Autodesk Inventor part; units mm, degrees
ref_plane "YZ Plane" through (0, 0, 0) normal (1, 0, 0) x (0, 1, 0)
ref_plane "XZ Plane" through (0, 0, 0) normal (0, 1, 0) x (-1, 0, 0)
ref_plane "XY Plane" through (0, 0, 0) normal (0, 0, 1) x (1, 0, 0)
sketch "Sketch1" plane through (0, 0, 0) normal (0, 0, 1) x (1, 0, 0)
  line L0 (-12.245, 11.65) -> (-12.245, 3)
  line L1 (-12.245, 3) -> (-45.245, 3)
  line L2 (-45.245, 3) -> (-45.245, 0)
  line L3 (-45.245, 0) -> (-10.245, 0)
  line L4 (-10.245, 0) -> (-10.245, 8.8)
  line L5 (-10.245, 8.8) -> (10.245, 8.8)
  line L6 (10.245, 8.8) -> (10.245, 0)
  line L7 (10.245, 0) -> (45.245, 0)
  line L8 (45.245, 0) -> (45.245, 3)
  line L9 (45.245, 3) -> (12.245, 3)
  line L10 (12.245, 3) -> (12.245, 11.65)
  line L11 (12.245, 11.65) -> (-12.245, 11.65)
  line L12 (-10.245, 0) -> (10.245, 0) construction
  point P0 (0, 0)
  point P1 (0, 11.65)
  point P2 (0, 0)
  point P3 (-12.245, 7.325)
  point P4 (12.245, 7.325)
  dimension "d0" = 20.49
  dimension "d1" = 2.85
  dimension "d3" = 5.8
  dimension "d4" = 3
  dimension "d5" = 3
  dimension "d6" = 35
  dimension "d7" = 35
  dimension "d73" = 33
  dimension "d74" = 33
extrude "Extrusion1" add sketch "Sketch1" along normal mid plane 41.1
sketch "Sketch8" plane through (12.245, 3, 20.55) normal (0, 1, 0) x (1, 0, 0)
  line L0 (0, 41.1) -> (0, 0)
  line L1 (33, 0) -> (0, 0)
  line L2 (33, 41.1) -> (33, 0)
  line L3 (0, 41.1) -> (33, 41.1)
  line L4 (-57.49, 41.1) -> (-57.49, 0)
  line L5 (-24.49, 0) -> (-57.49, 0)
  line L6 (-24.49, 0) -> (-24.49, 41.1)
  line L7 (-57.49, 41.1) -> (-24.49, 41.1)
  line L8 (33, 41.1) -> (33, 0)
  circle A0 centre (-11.645, 30.6) radius 6.4
  line L9 (-12.245, 41) -> (-12.245, 0) construction
  point P0 (-12.245, 20.55)
  point P1 (-54.49, 30.65)
  point P2 (-29.49, 30.65)
  point P3 (-57.49, 20.55)
  point P4 (30, 30.65)
  point P5 (5, 30.65)
  dimension "d42" = 3
  dimension "d43" = 25
  dimension "d51" = 10.45
  dimension "d53" = 3
hole "Hole1" at (-42.245, 3, -10.1) at (-17.245, 3, -10.1) at (17.245, 3, -10.1) at (42.245, 3, -10.1) direction (0, -1, 0) diameter 2.53 end through all
sketch "Sketch9" plane through (12.245, 3, 20.55) normal (0, 1, 0) x (1, 0, 0)
  circle A0 centre (30, 30.65) radius 1.265
  circle A1 centre (5, 30.65) radius 1.265
  line L0 (0, 41.1) -> (0, 0)
  line L1 (33, 0) -> (0, 0)
  line L2 (33, 41.1) -> (33, 0)
  line L3 (0, 41.1) -> (33, 41.1)
  arc A2 (33, 24) -> (9, 0) centre (33, 0) ccw
  point P0 (-12.245, 20.55)
  dimension "d60" = 24
extrude "Extrusion2" cut sketch "Sketch9" against normal blind 10 contours A2 L2 L1
mirror "Mirror1" about plane through (0, 0, 0) normal (1, 0, 0) of "Extrusion2"
sketch "Sketch10" plane through (-12.245, 11.65, 20.55) normal (0, 1, 0) x (1, 0, 0)
  circle A0 centre (12.245, 30.602) radius 6.5
  line L0 (0, 41.1) -> (0, 0)
  line L1 (24.49, 0) -> (0, 0)
  line L2 (24.49, 41.1) -> (24.49, 0)
  line L3 (0, 41.1) -> (24.49, 41.1)
  point P0 (12.245, 20.55)
  point P1 (12.245, 41.1)
  dimension "d75" = 13
  dimension "d76" = 10.498
extrude "Extrusion3" cut sketch "Sketch10" against normal blind 10 contours A0
sketch "Sketch11" plane through (-12.245, 11.65, 20.55) normal (0, 1, 0) x (1, 0, 0)
  circle A0 centre (5.245, 10.482) radius 0.7835
  circle A1 centre (4.245, 23.702) radius 0.7835
  circle A2 centre (4.175, 38.602) radius 0.7835
  circle A3 centre (20.315, 38.602) radius 0.7835
  circle A4 centre (20.245, 23.702) radius 0.7835
  circle A5 centre (19.245, 10.482) radius 0.7835
hole "Hole2" at (-8, 11.65, -3.152) at (8, 11.65, -3.152) at (8.07, 11.65, -18.052) at (-8.07, 11.65, -18.052) at (-7, 11.65, 10.068) at (7, 11.65, 10.068) direction (0, -1, 0) diameter 2.1 end through all counterbore diameter 4.1 counterbore depth 1.4
fillet "Fillet3" radius 3 6 edges at (45.245, 1.5, -20.55) (45.245, 1.5, -3.45) (21.245, 1.5, 20.55) (-21.245, 1.5, 20.55) (-45.245, 1.5, -3.45) (-45.245, 1.5, -20.55)
sketch "Sketch15" plane through (-10.245, 8.8, 20.55) normal (0, -1, 0) x (1, 0, 0)
  line L0 (0, -41.1) -> (0, 0)
  line L1 (20.49, -41.1) -> (20.49, 0)
  line L2 (0, -41.1) -> (0, -44.1)
  line L3 (0, -44.1) -> (20.49, -44.1)
  line L4 (20.49, -44.1) -> (20.49, -41.1)
  line L5 (0, 0) -> (0, 3)
  line L6 (0, 3) -> (20.49, 3)
  line L7 (20.49, 3) -> (20.49, 0)
  line L8 (0, -44.1) -> (0, 3)
  line L9 (20.49, 3) -> (20.49, -44.1)
  point P0 (10.245, -20.55)
  point P1 (0, 1.5)
  dimension "d126" = 3
  dimension "d127" = 3
sketch "Sketch16" plane through (-12.245, 11.65, 20.55) normal (0, 1, 0) x (1, 0, 0)
  line L0 (-30, 41.1) -> (0, 41.1)
  arc A0 (-30, 41.1) -> (-33, 38.1) centre (-30, 38.1) ccw
  line L1 (-33, 38.1) -> (-33, 26.8328)
  arc A1 (-33, 26.8328) -> (-30.3333, 23.8514) centre (-30, 26.8328) ccw
  arc A2 (-9.1486, 2.6667) -> (-30.3333, 23.8514) centre (-33, 0) ccw
  arc A3 (-9.1486, 2.6667) -> (-6.1672, 0) centre (-6.1672, 3) ccw
  line L2 (0, 0) -> (-6.1672, 0)
  line L3 (24.49, 0) -> (0, 0)
  line L4 (30.6572, 0) -> (24.49, 0)
  arc A4 (30.6572, 0) -> (33.6386, 2.6667) centre (30.6572, 3) ccw
  arc A5 (54.8233, 23.8514) -> (33.6386, 2.6667) centre (57.49, 0) ccw
  arc A6 (54.8233, 23.8514) -> (57.49, 26.8328) centre (54.49, 26.8328) ccw
  line L5 (57.49, 38.1) -> (57.49, 26.8328)
  arc A7 (57.49, 38.1) -> (54.49, 41.1) centre (54.49, 38.1) ccw
  line L6 (24.49, 41.1) -> (54.49, 41.1)
  line L7 (0, 41.1) -> (24.49, 41.1)
  point P0 (12.245, 20.55)
sketch "Sketch17" plane through (-12.245, 3, 20.55) normal (0, 1, 0) x (1, 0, 0)
  line L0 (0, 0) -> (0, 41.1)
  line L1 (-30, 41.1) -> (0, 41.1)
  arc A0 (-30, 41.1) -> (-33, 38.1) centre (-30, 38.1) ccw
  line L2 (-33, 38.1) -> (-33, 26.8328)
  arc A1 (-33, 26.8328) -> (-30.3333, 23.8514) centre (-30, 26.8328) ccw
  arc A2 (-9.1486, 2.6667) -> (-30.3333, 23.8514) centre (-33, 0) ccw
  arc A3 (-9.1486, 2.6667) -> (-6.1672, 0) centre (-6.1672, 3) ccw
  line L3 (0, 0) -> (-6.1672, 0)
  line L4 (30.6572, 0) -> (24.49, 0)
  arc A4 (30.6572, 0) -> (33.6386, 2.6667) centre (30.6572, 3) ccw
  arc A5 (54.8233, 23.8514) -> (33.6386, 2.6667) centre (57.49, 0) ccw
  arc A6 (54.8233, 23.8514) -> (57.49, 26.8328) centre (54.49, 26.8328) ccw
  line L5 (57.49, 38.1) -> (57.49, 26.8328)
  line L6 (24.49, 41.1) -> (54.49, 41.1)
  arc A7 (57.49, 38.1) -> (54.49, 41.1) centre (54.49, 38.1) ccw
  line L7 (24.49, 41.1) -> (24.49, 0)
  arc A8 (-36, 26.8328) -> (-30.6667, 20.87) centre (-30, 26.8328) ccw
  line L8 (-36, 26.8328) -> (-36, 38.1)
  arc A9 (-30, 44.1) -> (-36, 38.1) centre (-30, 38.1) ccw
  line L9 (-30, 44.1) -> (0, 44.1)
  line L10 (0, -3) -> (-6.1672, -3)
  arc A10 (-12.13, 2.3333) -> (-6.1672, -3) centre (-6.1672, 3) ccw
  arc A11 (-12.13, 2.3333) -> (-30.6667, 20.87) centre (-33, 0) ccw
  arc A12 (30.6572, -3) -> (36.62, 2.3333) centre (30.6572, 3) ccw
  line L11 (30.6572, -3) -> (24.49, -3)
  line L12 (24.49, 44.1) -> (54.49, 44.1)
  arc A13 (60.49, 38.1) -> (54.49, 44.1) centre (54.49, 38.1) ccw
  line L13 (60.49, 38.1) -> (60.49, 26.8328)
  arc A14 (55.1567, 20.87) -> (60.49, 26.8328) centre (54.49, 26.8328) ccw
  arc A15 (55.1567, 20.87) -> (36.62, 2.3333) centre (57.49, 0) ccw
  line L14 (0, 0) -> (0, -3)
  line L15 (0, 41.1) -> (0, 44.1)
  line L16 (24.49, 41.1) -> (24.49, 44.1)
  line L17 (24.49, 0) -> (24.49, -3)
  line L18 (0, 44.1) -> (0, -3)
  line L19 (24.49, -3) -> (24.49, 44.1)
  line L20 (-33, 38.1) -> (-33, 26.8328)
  point P0 (12.245, 20.55)
  dimension "d136" = 3
  dimension "d137" = 3
  dimension "d138" = 3
  dimension "d139" = 3
  dimension "d140" = 3
  dimension "d141" = 3
  dimension "d142" = 3
  dimension "d143" = 3
ref_plane "Work Plane1" through (0, 0, 0) normal (1, 0, 0) x (0, 1, 0)
properties part number "gripper_fixer"
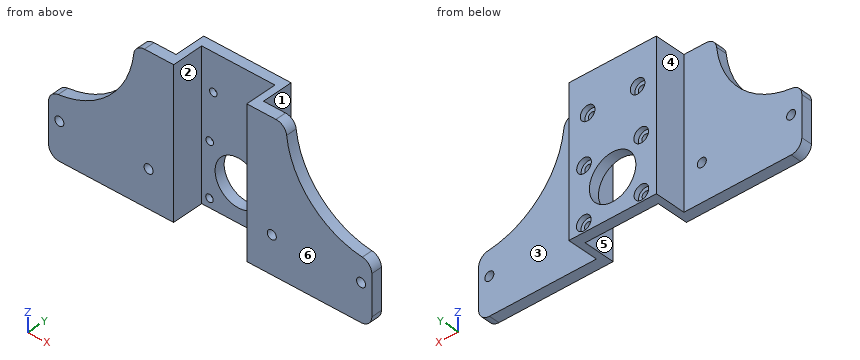
Source: CAD feature listing. Evaluate the final solid. Frame: model axes, mm. Face numbers are marked on the shaded views. A direction names the side the tool comes from. Give positions to 0.01 mm unless a question says otherwise; leave off trailing zeros. Write each loop counter-clockwise with the first axis right and the second up, starting at its lowest first coordinate (ties: lowest second). Pieces come first, ordered by that corner, then holes. Notation, with made-up numbers: (87.5, 44) - (119.5, 44) arc R14 cw to (119.5, 63) - close; hole circle Ø10 at (-28, -7). An arc over 180 degrees is marked (long way). Write item = value, one per line. Start each with the question number.
Q1. Reachability of the marked faces 4, 5 and 6 from +Z, -Z, +X, -X, +Y, -Y: full face, straight path, thin tool, end or side. Return the list, or none.
Q2. Cut plane C-C, the plane y = 1.75. Return loops of the section in (x, z) (3 decimals), then the cut area to 3 significant figures.
Q3. Draft query along X for the marked faces 1, 2 and 3. Return one class per face: +X half, -X half, draft (parallel to the pull), parting line (faces both ways), or undercut.
Q4. Cut plane D-D, the plane z = -8. Return loops of the section in (x, y) (3 decimals), then the cut area to 3 significant figures.
Q5. Cut plane A-A, the plane y = 7. Return loops of the section in (x, z) (3 decimals).
Q6. Material intervals for probe 1 along X at (y, z) = (0.9, -10.1) (3 decimals); probe 2 along X at (y, z) = (6.5, -7) (3 decimals); probe 3 along X at (y, z) = (10.75, -10.5) (3 decimals), sorted ascending.
Q7. Pin query (flat end, axial travel): pin 1 Ø2.5 at (y, z) = (3.5, -5) entering from +X; pin 2 Ø3.5 at (x, z) = (8, -3.152) entering from -Y; pin 3 Ø17 at (x, z) = (0, -10.052) entering from +Y; pin 4 Ø5 at (x, z) = (-31.5, -5) entering from +Y. Return the tip coordinate at first contact, or that it passes through.
Q8. Cut plane B-B, the plane x = 0. Return loops of the section in (y, z).
Computed values:
q1.face_4 = +Z, -Z, -X, +Y
q1.face_5 = +Z, -Z, -Y
q1.face_6 = +Z, -Z, +X, -X, -Y
q2.outline = (-45.245, -17.55) arc R3 ccw to (-42.245, -20.55) - (-10.245, -20.55) - (-10.245, 20.55) - (-18.412, 20.55) arc R3 ccw to (-21.394, 17.883) arc R24 cw to (-42.578, -3.301) arc R3 ccw to (-45.245, -6.283) - close; (10.245, -20.55) - (42.245, -20.55) arc R3 ccw to (45.245, -17.55) - (45.245, -6.283) arc R3 ccw to (42.578, -3.301) arc R24 cw to (21.394, 17.883) arc R3 ccw to (18.412, 20.55) - (10.245, 20.55) - close; hole circle Ø2.53 at (-42.245, -10.1); hole circle Ø2.53 at (-17.245, -10.1); hole circle Ø2.53 at (17.245, -10.1); hole circle Ø2.53 at (42.245, -10.1)
q2.area = 1,940 mm²
q3.face_1 = +X half
q3.face_2 = undercut
q3.face_3 = draft
q4.outline = (-45.245, 0) - (-10.245, 0) - (-10.245, 8.8) - (-6.168, 8.8) - (-6.168, 11.65) - (-12.245, 11.65) - (-12.245, 3) - (-45.245, 3) - close; (6.168, 8.8) - (10.245, 8.8) - (10.245, 0) - (45.245, 0) - (45.245, 3) - (12.245, 3) - (12.245, 11.65) - (6.168, 11.65) - close
q4.area = 268 mm²
q5.outline = (-12.245, -20.55) - (-10.245, -20.55) - (-10.245, 20.55) - (-12.245, 20.55) - close; (10.245, -20.55) - (12.245, -20.55) - (12.245, 20.55) - (10.245, 20.55) - close
q6.probe_1 = -45.245 to -43.51, -40.98 to -18.51, -15.98 to -10.245, 10.245 to 15.98, 18.51 to 40.98, 43.51 to 45.245
q6.probe_2 = -12.245 to -10.245, 10.245 to 12.245
q6.probe_3 = -12.245 to -6.485, 6.485 to 12.245
q7.pin_1 = 45.24
q7.pin_2 = 8.8
q7.pin_3 = 11.65
q7.pin_4 = 3
q8.outline = (8.8, -20.55) - (11.65, -20.55) - (11.65, -16.55) - (8.8, -16.55) - close; (8.8, -3.55) - (11.65, -3.55) - (11.65, 20.55) - (8.8, 20.55) - close
